Part model, mm, in its own coordinate system. Face numbers are marked on the shaded views. A direction names the side the tool comes from. Give positions to 0.01 mm unless a question says otherwise; leave off trailing zeros. Loops run counter-clockwise (first coordinate to the right, second up) from the corner with the lowest first, then second, coordinate; pieces in that order, holes last. Notation, with made-up numbers: M 43.25,-16 L 85.25,-16 A23 cw 85.25,10 Z; hole C 58.5,29 d3. An arc over 180 degrees is marked long. Answer in a Markdown table with one row per item.
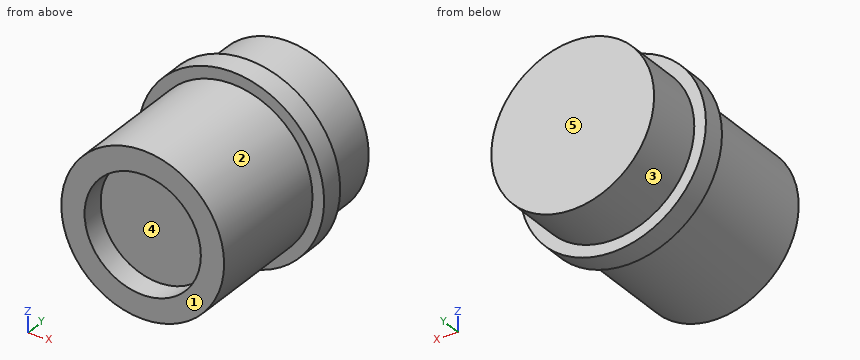
from build123d import *

# Parameters (mm, degrees)
SKETCH1_R                = 8
BOSS_EXTRUDE1_DEPTH      = 2
SKETCH2_R                = 7
BOSS_EXTRUDE2_DEPTH      = 5
BOSS_EXTRUDE2_DEPTH_BACK = 13
SKETCH4_R                = 5
CUT_EXTRUDE2_DEPTH       = 2


with BuildPart() as part:
    # Sketch1 → Boss-Extrude1 (new body)
    with BuildSketch(Plane(origin=(0, 0, 0), x_dir=(1, 0, 0), z_dir=(0, 1, 0))):
        Circle(SKETCH1_R)
    extrude(amount=BOSS_EXTRUDE1_DEPTH)

    # Sketch2 → Boss-Extrude2 (add, two sides)
    with BuildSketch(Plane(origin=(0, 2, 0), x_dir=(1, 0, 0), z_dir=(0, 1, 0))) as boss_extrude2_sk:
        Circle(SKETCH2_R)
    extrude(amount=BOSS_EXTRUDE2_DEPTH)
    extrude(boss_extrude2_sk.sketch, amount=-BOSS_EXTRUDE2_DEPTH_BACK)

    # Sketch4 → Cut-Extrude2 (cut)
    with BuildSketch(Plane.XZ.offset(11)):
        Circle(SKETCH4_R)
    extrude(amount=-CUT_EXTRUDE2_DEPTH, mode=Mode.SUBTRACT)


solid = part.part
(1) Saw through at C-C (y = -2). Write the cut outline in (x, z).
Recorded:
| item | result |
|---|---|
| outline | C 0,0 d14 |
(2) Pin check, flat tips, straight feed: pin 1 Ø3 at (x, z) = (0.5, -2) entering from -Y; pin 2 Ø1.5 at (x, y) = (-4.5, 4) entering from -Z; pin 3 Ø8 at (x, z) = (-4.5, 5.5) entering from -Y; pin 4 Ø4 at (x, y) = (5.5, 0.5) entering from -Z. Stop position of each tip, or through.
Recorded:
| item | result |
|---|---|
| pin 1 | stops at y = -9 |
| pin 2 | stops at z = -5.91 |
| pin 3 | stops at y = -11 |
| pin 4 | stops at z = -7.19 |
(3) Drill centre lines: line 1 along Y through (x, z) = (5.75, 5.25); line 2 along Y through (x, z) = (0.25, 2.5); line 3 along Z through (x, y) = (0, -9.7). Where is each one in solid material? Low to high.
Recorded:
| item | result |
|---|---|
| line 1 | y = 0 to 2 |
| line 2 | y = -9 to 7 |
| line 3 | z = -7 to -5, 5 to 7 |
(4) Pull direction X, two halves, no side cores. Call the marked faces 3, 4 and 5: +X half, -X half, draft (parallel to the pull), parting line (faces both ways), or undercut.
Recorded:
| item | result |
|---|---|
| face 3 | parting line |
| face 4 | undercut |
| face 5 | draft |
(5) Saw through at B-B (x = 0). Write the cut outline in (y, z).
Recorded:
| item | result |
|---|---|
| outline | M -11,-7 L 0,-7 L 0,-8 L 2,-8 L 2,-7 L 7,-7 L 7,7 L 2,7 L 2,8 L 0,8 L 0,7 L -11,7 L -11,5 L -9,5 L -9,-5 L -11,-5 Z |
(6) Saw through at D-D (y = 1). Write the cut outline in (x, z), plus the area to 3 significant figures.
Recorded:
| item | result |
|---|---|
| outline | C 0,0 d16 |
| area | 201 mm^2 |
(7) Which spindle directions (+Z, -Z, +X, -X, +Y, -Y) get a long thin tool onto all of the face, cutting with end or side? Do the marked faces 1 and 2. Say none if no direction does.
Recorded:
| item | result |
|---|---|
| face 1 | +Z, -Z, +X, -X, -Y |
| face 2 | -Y |
(8) Saw through at A-A (z = 0). Write the cut outline in (x, y).
Recorded:
| item | result |
|---|---|
| outline | M -8,0 L -7,0 L -7,-11 L -5,-11 L -5,-9 L 5,-9 L 5,-11 L 7,-11 L 7,0 L 8,0 L 8,2 L 7,2 L 7,7 L -7,7 L -7,2 L -8,2 Z |
